Input: part model. Units: mm. Frame: model coordinates. Face numbers are marked on the shaded views. A direction names the side the tool comes from. Give positions to 0.01 mm unless a question says otherwise; leave off trailing zeros. Loops run counter-clockwise (first coordinate to the right, second up) from the corner with the lowest first, then second, coordinate; pieces in that order, holes last. Notation, with made-up numbers: (63, -31) - (113, -31) arc R25 ccw to (113, -2) - close; hole circle Ø4 at (77, 41). An arc over 180 degrees is marked (long way). One line per item, written item: value.
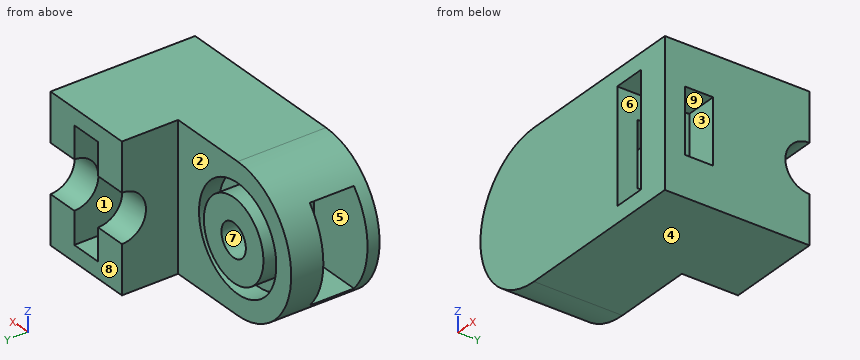
from build123d import *

# Parameters (mm, degrees)
SKETCH2_W               = 11
SKETCH2_H               = 9
BOSS_EXTRUDE1_DEPTH     = 9
SKETCH3_W               = 15.859827236
SKETCH3_H               = 9.999542671
CUT_EXTRUDE1_DEPTH      = 3.5
CUT_EXTRUDE2_DEPTH      = 13.5
SKETCH5_W               = 2
SKETCH5_H               = 7
CUT_EXTRUDE3_DEPTH      = 28.773973587
SKETCH6_R               = 3.25
CUT_EXTRUDE4_DEPTH      = 1.25
SKETCH7_R               = 2.5
BOSS_EXTRUDE2_DEPTH     = 1.5
SKETCH8_W               = 4
SKETCH8_H               = 1.75
CUT_EXTRUDE5_DEPTH      = 21.5
SKETCH9_W               = 6
SKETCH9_H               = 2.75
CUT_EXTRUDE6_DEPTH      = 4.5
M2_5_TAPPED_HOLE2_D     = 2.05
M2_5_TAPPED_HOLE2_DEPTH = 3
M2_5_TAPPED_HOLE2_TIP   = 0.615882135
SKETCH11_W              = 2.05
SKETCH11_H              = 0.5
BOSS_EXTRUDE3_DEPTH     = 4


with BuildPart() as part:
    # Sketch2 → Boss-Extrude1 (new body)
    with BuildSketch(Plane(origin=(0, 0, 0), x_dir=(1, 0, 0), z_dir=(0, 1, 0))):
        with BuildLine():
            Line((-5.5, -4.5), (-5.5, 4.5))
            ThreePointArc((-5.5, 4.5), (-10, 0), (-5.5, -4.5))
        make_face()
        Rectangle(SKETCH2_W, SKETCH2_H)
    extrude(amount=BOSS_EXTRUDE1_DEPTH)

    # Sketch3 → Cut-Extrude1 (cut)
    with BuildSketch(Plane(origin=(0, 9, 0), x_dir=(1, 0, 0), z_dir=(0, 1, 0))):
        with Locations((-8.429913618, -0.499771336)):
            Rectangle(SKETCH3_W, SKETCH3_H)
    extrude(amount=-CUT_EXTRUDE1_DEPTH, mode=Mode.SUBTRACT)

    # Sketch4 → Cut-Extrude2 (cut)
    with BuildSketch(Plane.ZY.offset(0.5)):
        with BuildLine():
            Line((-1.5, 9), (1.5, 9))
            ThreePointArc((1.5, 9), (0, 7.5), (-1.5, 9))
        make_face()
    extrude(amount=-CUT_EXTRUDE2_DEPTH, mode=Mode.SUBTRACT)

    # Sketch5 → Cut-Extrude3 (cut)
    with BuildSketch(Plane(origin=(0, 9, 0), x_dir=(1, 0, 0), z_dir=(0, 1, 0))):
        with Locations((2.5, 0)):
            Rectangle(SKETCH5_W, SKETCH5_H)
    extrude(amount=-CUT_EXTRUDE3_DEPTH, mode=Mode.SUBTRACT)

    # Sketch6 → Cut-Extrude4 (cut)
    with BuildSketch(Plane(origin=(0, 5.5, 0), x_dir=(1, 0, 0), z_dir=(0, 1, 0))):
        with Locations((-5.5, 0)):
            Circle(SKETCH6_R)
    extrude(amount=-CUT_EXTRUDE4_DEPTH, mode=Mode.SUBTRACT)

    # Sketch7 → Boss-Extrude2 (add)
    with BuildSketch(Plane(origin=(0, 4.25, 0), x_dir=(1, 0, 0), z_dir=(0, 1, 0))):
        with Locations((-5.5, 0)):
            Circle(SKETCH7_R)
    extrude(amount=BOSS_EXTRUDE2_DEPTH)

    # Sketch8 → Cut-Extrude5 (cut)
    with BuildSketch(Plane(origin=(5.5, 0, 0), x_dir=(0, 0, -1), z_dir=(1, 0, 0))):
        with Locations((0, 2.125)):
            Rectangle(SKETCH8_W, SKETCH8_H)
    extrude(amount=-CUT_EXTRUDE5_DEPTH, mode=Mode.SUBTRACT)

    # Sketch9 → Cut-Extrude6 (cut)
    with BuildSketch(Plane(origin=(-10, 0, 0), x_dir=(0, 0, -1), z_dir=(1, 0, 0))):
        with Locations((0, 2.125)):
            Rectangle(SKETCH9_W, SKETCH9_H)
    extrude(amount=CUT_EXTRUDE6_DEPTH, mode=Mode.SUBTRACT)

    # M2.5 Tapped Hole2
    with Locations(Plane(origin=(-5.5, 5.75, 0), x_dir=(0, 0, 1), z_dir=(0, 1, 0))):
        with Locations((0, 0)):
            Hole(M2_5_TAPPED_HOLE2_D / 2, depth=M2_5_TAPPED_HOLE2_DEPTH)
            with Locations((0, 0, -(M2_5_TAPPED_HOLE2_DEPTH + M2_5_TAPPED_HOLE2_TIP / 2))):  # 118° drill point
                Cone(0, M2_5_TAPPED_HOLE2_D / 2, M2_5_TAPPED_HOLE2_TIP, mode=Mode.SUBTRACT)

    # Sketch11 → Boss-Extrude3 (add)
    with BuildSketch(Plane.ZY.offset(5.5)):
        with Locations((0, 3.25)):
            Rectangle(SKETCH11_W, SKETCH11_H)
    extrude(amount=-BOSS_EXTRUDE3_DEPTH)


solid = part.part
Item 1: Access query for the marked faces 5, 6, 7, 8 and 9. Directions: +Z, -Z, +X, -X, +Y, -Y. A direction counts if a zero-diameter tool reaches every point of the face in a straight line with its end or side. Return the directions, or none.
Verdict:
face 5: -X
face 6: +Y, -Y
face 7: +Y
face 8: +Z, -Z, +X, -X, +Y
face 9: +X, -X
Item 2: Section C-C, the plane y = 8. Output: boundary loops of the cut face in (x, z).
Verdict:
outline: (-0.5, -4.5) - (5.5, -4.5) - (5.5, -1.12) - (3.5, -1.12) - (3.5, -3.5) - (1.5, -3.5) - (1.5, -1.12) - (-0.5, -1.12) - close; (-0.5, 1.12) - (1.5, 1.12) - (1.5, 3.5) - (3.5, 3.5) - (3.5, 1.12) - (5.5, 1.12) - (5.5, 4.5) - (-0.5, 4.5) - close
Item 3: Section D-D, the plane z = -2.75. Output: boundary loops of the cut face in (x, y), and give its area (3 significant figures).
Verdict:
outline: (-9.06, 0) - (1.5, 0) - (1.5, 9) - (-0.5, 9) - (-0.5, 5.5) - (-3.77, 5.5) - (-3.77, 4.25) - (-7.23, 4.25) - (-7.23, 5.5) - (-9.06, 5.5) - (-9.06, 3.5) - (-5.5, 3.5) - (-5.5, 0.75) - (-9.06, 0.75) - close; (3.5, 0) - (5.5, 0) - (5.5, 9) - (3.5, 9) - close
area: 69.0 mm^2
Item 4: Pin query (flat end, axial travel): P1, Ø3, axis at y = 3.5, z = 2.5, coming from the -X side; P2, Ø2, axis at x = -7.5, y = 2.5, coming from the +Z side; P3, Ø2, axis at x = -2.5, z = -1.5, coming from the +Y side. Return the tip coordinate at first contact, or that it passes through.
Verdict:
P1: stops at x = -9.89
P2: stops at z = 4.39
P3: stops at y = 5.75
Item 5: Material intervals for L1, parallel to X at y = 4.75, z = 0 (3 decimals); L2, parallel to Z at x = -5.5, y = 4.3 (3 decimals); L3, parallel to X at y = 4.1, z = 0 (3 decimals), sorted ascending.
Verdict:
L1: x = -10 to -8.75, -8 to -6.525, -4.475 to -3, -2.25 to 1.5, 3.5 to 5.5
L2: z = -4.5 to -3.25, -2.5 to -1.025, 1.025 to 2.5, 3.25 to 4.5
L3: x = -10 to -6.525, -4.475 to 1.5, 3.5 to 5.5
Item 6: Section B-B, the plane x = 2. Output: boundary loops of the cut face in (y, z), and give its area (3 significant figures).
Verdict:
outline: (0, -4.5) - (9, -4.5) - (9, -3.5) - (0, -3.5) - close; (0, 3.5) - (9, 3.5) - (9, 4.5) - (0, 4.5) - close
area: 18.0 mm^2
Item 7: Section A-A, the plane z = 0. Count the separate pieces of the cut face and the enclosed holes in it, and give its area (3 significant figures).
Verdict:
separate pieces: 5
enclosed holes: 0
area: 48.9 mm^2
Item 8: Draft query along Z for the marked faces 1, 2, 3 and 4. Return one class per face: pulls with the +Z half, pulls with the -Z half, needs draft (parallel to the pull), parting line crosses it, or undercut.
Verdict:
face 1: undercut
face 2: needs draft
face 3: undercut
face 4: pulls with the -Z half
